Model file for the job. Use its own axes, mm. Round coordinates to 2 decimals unless told otherwise and drop trailing zeros. Order: outer loops, then holes, each group sorted by start corner. A loop starts at its lowest first (then second) coordinate and runs counter-clockwise, first axis right, second up. Notation, with made-up numbers: (-16, -24) -> (-3, -24) arc R17 ccw to (-3, 2) -> close; hole circle Ø7 at (57, 54.25). An arc over 180 degrees is marked (long way). Answer as CSV lines item,"result".
Autodesk Inventor part; units mm, degrees
ref_plane "YZ Plane" through (0, 0, 0) normal (1, 0, 0) x (0, 1, 0)
ref_plane "XZ Plane" through (0, 0, 0) normal (0, 1, 0) x (-1, 0, 0)
ref_plane "XY Plane" through (0, 0, 0) normal (0, 0, 1) x (1, 0, 0)
sketch "Sketch3" plane through (0, 0, 0) normal (0, 1, 0) x (-1, 0, 0)
  line L0 (0, 0) -> (67.5, 0)
  line L1 (0, 0) -> (0, 45)
  line L2 (67.5, 31.5278) -> (67.5, -31.5278)
  line L3 (0, 45) -> (54.1779, 45)
  line L4 (-67.5, 31.5278) -> (-67.5, -31.5278)
  line L5 (0, 45) -> (-54.1779, 45)
  arc A0 (67.5, 31.5278) -> (62.5776, 40.4264) centre (0, 0) ccw
  arc A1 (-62.5776, 40.4264) -> (-67.5, 31.5278) centre (0, 0) ccw
  arc A2 (-67.5, -31.5278) -> (67.5, -31.5278) centre (0, 0) ccw
  arc A3 (62.5776, 40.4264) -> (54.1779, 45) centre (54.1779, 35) ccw
  arc A4 (-54.1779, 45) -> (-62.5776, 40.4264) centre (-54.1779, 35) ccw
  point P0 (59.3738, 45)
  point P1 (-59.3738, 45)
  dimension "d28" = 67.5
  dimension "d29" = 45
  dimension "d30" = 10
  dimension "d31" = 10
  dimension "d32" = 74.5
  dimension "d34" = 67.5
  dimension "d35" = 74.5
extrude "Extrusion2" add sketch "Sketch3" along normal blind 2.7
properties part number "tapa_carcasa_4.0"
Q1. Saw through at B-B (x = 26.5). Write the cut outline in (y, z).
Checks:
outline,"(0, -69.63) -> (2.7, -69.63) -> (2.7, 45) -> (0, 45) -> close"
Q2. Saw through at C-C (z = -40). Write the cut outline in (x, y), plus the area to 3 significant figures.
Checks:
outline,"(-62.85, 0) -> (62.85, 0) -> (62.85, 2.7) -> (-62.85, 2.7) -> close"
area,"339 mm²"
Q3. Wall check: L1, parallel to Z at x = -1, y = 1.75; L2, parallel to Z at x = -31, y = 1.6; L3, parallel to X at y = 1.1, z = -56.5. Give the ranges that are in metal, low to high. Write a range as [from, to].
Checks:
L1,"[-74.49, 45]"
L2,"[-67.74, 45]"
L3,"[-48.56, 48.56]"
Q4. Saw through at A-A (y = 0.6). Write the cut outline in (x, z), plus the area to 3 significant figures.
Checks:
outline,"(-67.5, -31.53) arc R74.5 ccw to (67.5, -31.53) -> (67.5, 31.53) arc R74.5 ccw to (62.58, 40.43) arc R10 ccw to (54.18, 45) -> (-54.18, 45) arc R10 ccw to (-62.58, 40.43) arc R74.5 ccw to (-67.5, 31.53) -> close"
area,"14,400 mm²"
